Geometry check sheet. Reference: the model listing, model coordinates, mm. Give positions to 0.01 mm unless a question says otherwise; leave off trailing zeros. Write each loop counter-clockwise with the first axis right and the second up, starting at its lowest first coordinate (ties: lowest second). Pieces come first, ordered by that corner, then holes. Notation, with made-up numbers: (7.5, 72) - (13.5, 72) arc R18 cw to (13.5, 77) - close; hole circle Ø1 at (8.5, 59). An arc over 180 degrees is marked (long way). Use a Markdown table: item, result.
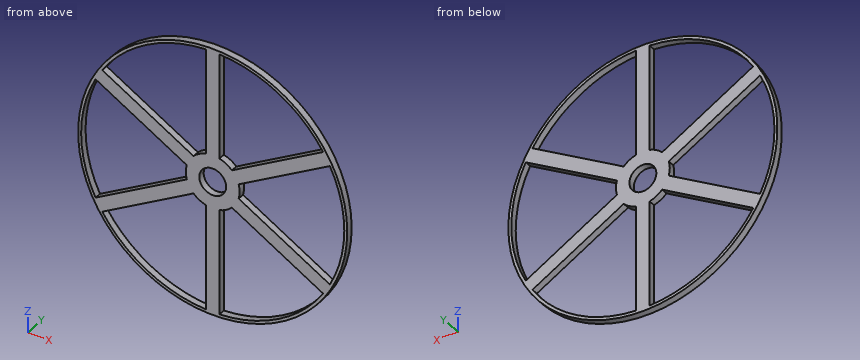
```python
from build123d import *

# Parameters (mm, degrees)
F0_R     = 31.75
F1_DEPTH = 1.5875
F2_R     = 3.175
F3_DEPTH = 25.4


with BuildPart() as f1:
    # F0 (on Front) → F1 (new body)
    with BuildSketch(Plane.XZ):
        Circle(F0_R)
        with BuildLine():
            Line((-26.062471, -16.880262), (-4.530887, -4.448996))
            ThreePointArc((-4.530887, -4.448996), (-3.175, -5.499261), (-1.5875, -6.148361))
            Line((-1.5875, -6.148361), (-1.5875, -31.010893))
            ThreePointArc((-1.5875, -31.010893), (-15.52575, -26.891388), (-26.062471, -16.880262))
        make_face(mode=Mode.SUBTRACT)
        with BuildLine():
            ThreePointArc((1.5875, -6.148361), (3.175, -5.499261), (4.530887, -4.448996))
            Line((4.530887, -4.448996), (26.062471, -16.880262))
            ThreePointArc((26.062471, -16.880262), (15.52575, -26.891388), (1.5875, -31.010893))
            Line((1.5875, -31.010893), (1.5875, -6.148361))
        make_face(mode=Mode.SUBTRACT)
        with BuildLine():
            ThreePointArc((6.118387, -1.699365), (6.35, 0), (6.118387, 1.699365))
            Line((6.118387, 1.699365), (27.649971, 14.130631))
            ThreePointArc((27.649971, 14.130631), (31.0515, 0), (27.649971, -14.130631))
            Line((27.649971, -14.130631), (6.118387, -1.699365))
        make_face(mode=Mode.SUBTRACT)
        with BuildLine():
            ThreePointArc((-6.118387, 1.699365), (-6.35, 0), (-6.118387, -1.699365))
            Line((-6.118387, -1.699365), (-27.649971, -14.130631))
            ThreePointArc((-27.649971, -14.130631), (-31.0515, 0), (-27.649971, 14.130631))
            Line((-27.649971, 14.130631), (-6.118387, 1.699365))
        make_face(mode=Mode.SUBTRACT)
        with BuildLine():
            ThreePointArc((-26.062471, 16.880262), (-15.52575, 26.891388), (-1.5875, 31.010893))
            Line((-1.5875, 31.010893), (-1.5875, 6.148361))
            ThreePointArc((-1.5875, 6.148361), (-3.175, 5.499261), (-4.530887, 4.448996))
            Line((-4.530887, 4.448996), (-26.062471, 16.880262))
        make_face(mode=Mode.SUBTRACT)
        with BuildLine():
            ThreePointArc((4.530887, 4.448996), (3.175, 5.499261), (1.5875, 6.148361))
            Line((1.5875, 6.148361), (1.5875, 31.010893))
            ThreePointArc((1.5875, 31.010893), (15.52575, 26.891388), (26.062471, 16.880262))
            Line((26.062471, 16.880262), (4.530887, 4.448996))
        make_face(mode=Mode.SUBTRACT)
    extrude(amount=F1_DEPTH)

    # F2 (on face) → F3 (cut)
    with BuildSketch(Plane.XZ.offset(1.5875)):
        Circle(F2_R)
    extrude(amount=-F3_DEPTH, mode=Mode.SUBTRACT)


solid = f1.part
```
1) Material ranges on L1, parallel to Z at x = 0, y = -0.4 (3 decimals); L2, parallel to Z at x = -25, y = -0.1; L3, parallel to Z at x = 5.5, y = -0.8, recorded low to high. Write a range as from..to.
Working result:
| item | result |
|---|---|
| L1 | z = -31.75..-3.175, 3.175..31.75 |
| L2 | z = -19.57..-18.42, -16.27..-12.6, 12.6..16.27, 18.42..19.57 |
| L3 | z = -31.27..-30.56, -5.01..5.01, 30.56..31.27 |
2) Section check A-A on z = 0. Count the separate pieces of the cut face and the enclosed holes in it, then the cut area to 3 significant figures.
Working result:
| item | result |
|---|---|
| separate pieces | 4 |
| enclosed holes | 0 |
| area | 12.3 mm² |
3) Depth check by flat-ended pin: P1, Ø5.5, axis at x = 0, z = 0, coming from the -Y side; P2, Ø0.8, axis at y = -1, z = 16.5, coming from the +X side; P3, Ø0.8, axis at y = -1, z = -13, coming from the +X side; P4, Ø0.8, axis at y = -1, z = -23.5, coming from the -X side. Enter the tip coordinate at first touch or a pass-through.
Working result:
| item | result |
|---|---|
| P1 | passes through |
| P2 | stops at x = 27.37 |
| P3 | stops at x = 29.14 |
| P4 | stops at x = -21.78 |
4) Section check D-D on x = 15.5. Record the boundary of the cut face in (y, z), then the cut area to 3 significant figures.
Working result:
| item | result |
|---|---|
| outline | (-1.59, -27.71) - (0, -27.71) - (0, -26.91) - (-1.59, -26.91) - close; (-1.59, -10.78) - (0, -10.78) - (0, -7.12) - (-1.59, -7.12) - close; (-1.59, 7.12) - (0, 7.12) - (0, 10.78) - (-1.59, 10.78) - close; (-1.59, 26.91) - (0, 26.91) - (0, 27.71) - (-1.59, 27.71) - close |
| area | 14.2 mm² |
